The model under review builds one solid part; all positions refer to its coordinate system, in mm. Face numbers are marked on the shaded views. Give positions to 0.01 mm unless a question says otherwise; leave off trailing zeros. Order: outer loops, then holes, each group sorted by start corner. A loop starts at its lowest first (then second) coordinate and runs counter-clockwise, first axis right, second up. Notation, with made-up numbers: (30, 41) - (84, 41) arc R24 ccw to (84, 80) - close; hole circle Ø6 at (-20.75, 23). An arc over 180 degrees is marked (long way). Write item = value, one per line. Start each with the question number.
1. Wall thickness on probe 1 along Z at (x, y) = (0, 23.75); probe 2 along X at (y, z) = (24.75, -150); probe 3 along Z at (x, y) = (-2, 25.25): over which ranges is each line inside the solid? List them lowest first.
2. For P1, Ø8, axis at x = 75.5, z = 141.5, coming from the +Y side; P2, Ø5.5, axis at x = -2, z = -151, coming from the +Y side, all flat-tipped, find the tip position at first contact; note any pin that passes through.
3. We need section B-B, the plane z = 172.5. Give the boundary of the cut face in (x, y).
4. Mouldability with a two-part tool opening along X and no side actions: class the marked faces 1 and 2 as pulls with the +X half, pulls with the -X half, needs draft (parallel to the pull), parting line crosses it, or undercut.
5. We need section A-A, the plane x = 91. Give the boundary of the cut face in (y, z), and give its area (3 significant figures).
Autodesk Inventor part; units mm, degrees
ref_plane "YZ Plane" through (0, 0, 0) normal (1, 0, 0) x (0, 1, 0)
ref_plane "XZ Plane" through (0, 0, 0) normal (0, 1, 0) x (-1, 0, 0)
ref_plane "XY Plane" through (0, 0, 0) normal (0, 0, 1) x (1, 0, 0)
sketch "Sketch1" plane through (0, 0, 0) normal (0, 1, 0) x (-1, 0, 0)
  line L0 (105, -200) -> (-105, -200)
  line L1 (-105, -200) -> (-105, 200)
  line L2 (-105, 200) -> (105, 200)
  line L3 (105, 200) -> (105, -200)
  line L4 (105, -200) -> (-105, 200) construction
  line L5 (-105, -200) -> (105, 200) construction
  point P0 (0, 0)
  dimension "d0" = 210
  dimension "d1" = 400
extrude "Extrusion1" add sketch "Sketch1" along normal blind 30
sketch "Sketch2" plane through (0, 30, 0) normal (0, 1, 0) x (1, 0, 0)
  circle A0 centre (0, 150) radius 9
  circle A1 centre (0, -150) radius 9
  line L0 (-105, -200) -> (105, -200)
  line L1 (105, 200) -> (-105, 200)
  point P0 (0, 0)
  dimension "d4" = 18
  dimension "d5" = 18
  dimension "d6" = 150
  dimension "d7" = 150
  dimension "d23" = 400
hole "Hole1" at (0, 30, -150) at (0, 30, 150) direction (0, -1, 0) diameter 0.1 end through all counterbore diameter 18 counterbore depth 24
sketch "Sketch3" plane through (0, 30, 0) normal (0, 1, 0) x (1, 0, 0)
  line L0 (65, -195) -> (100, -195)
  line L1 (100, -195) -> (100, -135)
  line L2 (100, -135) -> (65, -135)
  line L3 (65, -135) -> (65, -195)
  line L4 (-105, -200) -> (105, -200)
  line L5 (105, -200) -> (105, 200)
  point P0 (0, 0)
  dimension "d15" = 35
  dimension "d16" = 60
  dimension "d17" = 5
  dimension "d19" = 5
extrude "Extrusion2" cut sketch "Sketch3" against normal blind 3.5
fillet "Fillet1" radius 4 4 edges at (105, 15, 200) (-105, 15, 200) (105, 15, -200) (-105, 15, -200)
properties part number "Podstawa"
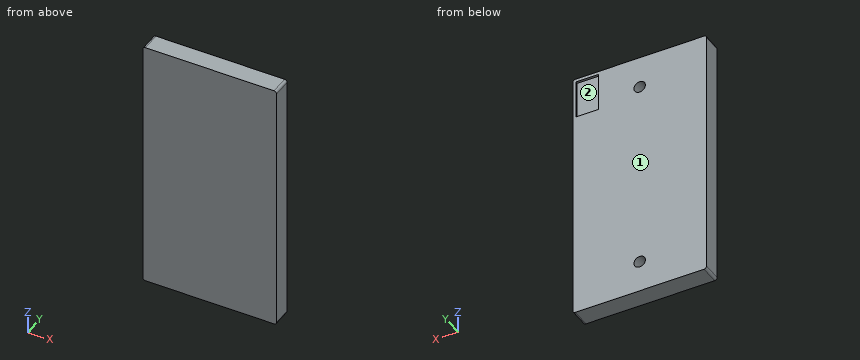
Model answer:
q1.probe_1 = -200 to -159, -141 to 141, 159 to 200
q1.probe_2 = -105 to -9, 9 to 105
q1.probe_3 = -200 to -158.77, -141.23 to 141.23, 158.77 to 200
q2.P1 = 26.5
q2.P2 = 6
q3.outline = (-105, 0) - (105, 0) - (105, 30) - (100, 30) - (100, 26.5) - (65, 26.5) - (65, 30) - (-105, 30) - close
q4.face_1 = needs draft
q4.face_2 = undercut
q5.outline = (0, -200) - (30, -200) - (30, 135) - (26.5, 135) - (26.5, 195) - (30, 195) - (30, 200) - (0, 200) - close
q5.area = 11,800 mm2
